Solid Edge part; units mm, degrees
sketch "Sketch1" plane through (0, 0, 0) normal (0, 0, 1) x (1, 0, 0)
  line L0 (3, 0) -> (3, 10)
  line L1 (0, 10) -> (3, 10)
  line L2 (0, 0) -> (0, 10)
  line L3 (0, 0) -> (0, -3.3)
  line L4 (0, -3.3) -> (5.25, -3.3)
  line L5 (5.25, -3.3) -> (5.25, 0)
  line L6 (5.25, 0) -> (3, 0)
revolve "RevolvedProtrusion1" add sketch "Sketch1" angle 360 about axis through (0, 0, 0) along (0, 1, 0)
sketch "Sketch2" plane through (0, 0, 0) normal (1, 0, 0) x (0, 1, 0)
  line L0 (-3.3, 2.7915) -> (-1.22, 2.7915)
  line L1 (0.3917, 0) -> (-1.22, 2.7915)
  line L2 (-3.3, 0) -> (0.3917, 0)
  line L3 (-3.3, 0) -> (-3.3, 2.7915)
revolve "RevolvedCutout1" cut sketch "Sketch2" angle 360 about axis through (0, -3.3, 0) along (0, 1, 0)
sketch "Sketch3" plane through (0, -3.3, 0) normal (0, -1, 0) x (0, 0, 1)
  circle A0 centre (0, 0) radius 2.7915
  line L0 (-2, -1.1547) -> (0, -2.3094)
  line L1 (0, -2.3094) -> (2, -1.1547)
  line L2 (2, -1.1547) -> (2, 1.1547)
  line L3 (2, 1.1547) -> (0, 2.3094)
  line L4 (0, 2.3094) -> (-2, 1.1547)
  line L5 (-2, 1.1547) -> (-2, -1.1547)
extrude "Protrusion1" add sketch "Sketch3" against normal up to next
sketch "Sketch4" plane through (0, 0, 0) normal (0, 0, 1) x (1, 0, 0)
  line L0 (-2.3094, -3.3) -> (0, -3.3)
  line L1 (0, -3.3) -> (0, -2.6812)
  line L2 (0, -2.6812) -> (-2.3094, -3.3)
revolve "RevolvedCutout2" cut sketch "Sketch4" angle 360 about axis through (0, -3.3, 0) along (0, 1, 0)
fillet "Round1" radius 0.25 1 edges at (0, 0, -3)
chamfer "倒斜角_2" distance 0.4 angle 45 1 edges at (0, 10, -3)
cosmetic_thread "螺纹_3" thread depth 8
sketch "Sketch5" plane through (0, 0, 0) normal (0, 0, 1) x (1, 0, 0)
  arc A0 (-3.0553, -3.3) -> (-5.25, 0) centre (-1.6717, 0) cw
revolve "RevolvedCutout3" cut sketch "Sketch5" angle 360 about axis through (0, 0, 0) along (0, -1, 0) material side at (-4.6929, -2.0093, 0)
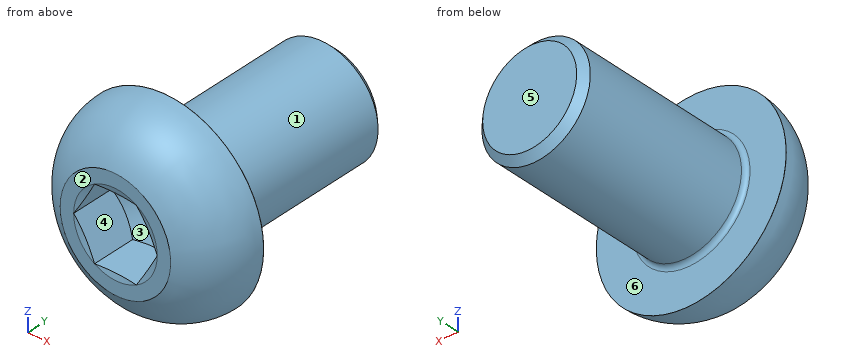
Could you check a few things on this model? Use its own coordinates, in mm. Face numbers are marked on the shaded views. A direction names the side the tool comes from. Round coordinates to 2 decimals unless told otherwise and drop trailing zeros. Loops run counter-clockwise (first coordinate to the right, second up) from the corner with the lowest first, then second, coordinate; pieces in that order, holes last.
Q1. Please list where these lines run through material, in increasing order: L1, parallel to Z at x = 0, y = 2.75; L2, parallel to Y at x = -3.5, z = 2; L3, parallel to Y at x = 3, z = 0.75.
Q2. Thinking about a two-plate mould opening in Z: for the marked faces 1, 2 and 3, which applies, pulls with the +Z half, pulls with the -Z half, needs draft (parallel to the pull), parting line crosses it, or undercut?
Q3. On a 3-axis mill with a long thin cutter (end or side, diameter ignored), from which of +Z, -Z, +X, -X, +Y, -Y can I reach the whole of each face in a straight line? I mean the marked faces 4, 5 and 6. Say none if no direction works.
Q4. For P1, Ø1.8, axis at x = 0, y = -2, coming from the -Z side; P2, Ø2, axis at y = 7, z = -2.5, coming from the -X side; P3, Ø2.5, axis at x = 0, y = -2, coming from the +Z side, each with a flat end and sliding along its axis, tell me the tip position at first contact or that it passes through.
Q5. I want a section at A-A (y = 5.5). Write out the boundary of the cut face in (x, z).
Answer below:
1. L1: z = -3 to 3
1. L2: y = -2.69 to 0
1. L3: y = -3.28 to 0.06
2. face 1: parting line crosses it
2. face 2: needs draft
2. face 3: undercut
3. face 4: -Y
3. face 5: +Z, -Z, +X, -X, +Y
3. face 6: +Y
4. P1: stops at z = -5.08
4. P2: stops at x = -2.6
4. P3: stops at z = 5.17
5. outline: circle Ø6 at (0, 0)
